Part model, mm, in its own coordinate system. Face numbers are marked on the shaded views. Round coordinates to 2 decimals unless told otherwise and drop trailing zeros. Loops run counter-clockwise (first coordinate to the right, second up) from the corner with the lowest first, then second, coordinate; pieces in that order, holes last. Notation, with made-up numbers: M 15.5,-4 L 43.5,-4 A23 ccw 43.5,14 Z; hole C 38,57 d6. An arc over 180 degrees is marked long. Answer as CSV lines item,"result". Start each with the question number.
Item 1: Drop a flat-ended pin along its axis: pin 1 Ø1.5 at (y, z) = (-2, 43.5) entering from -X. Give the stop position or say it passes through.
Item 2: Wall check: line 1 (Z direction, x = 17.5, y = -1.1); line 2 (Z direction, x = 16.25, y = -2.35); line 3 (X direction, y = -2.4, z = 23). Give the ranges that are in metal, low to high.
Item 3: Band-saw the part on A-A (y = -2.1). Give the cut face in (x, z).
Item 4: Mould opens along Y. For the marked faces 1 and 2 say: pulls with the +Y half, pulls with the -Y half, needs draft (parallel to the pull), parting line crosses it, or undercut.
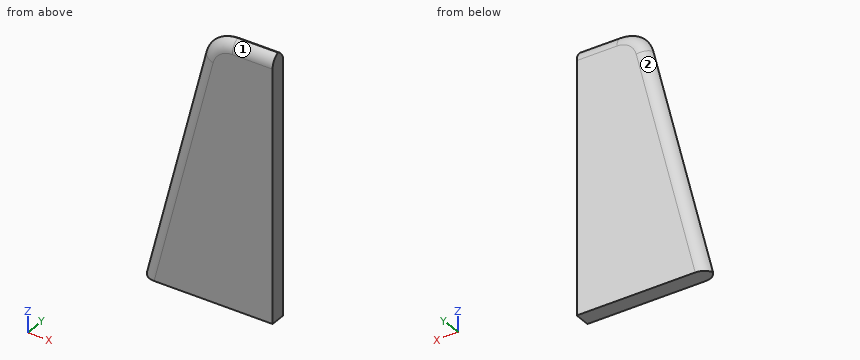
```python
from build123d import *

# Parameters (mm, degrees)
F1_DEPTH    = 3.048
F2_T1_DEPTH = 53.7555112647
F2_T3_DEPTH = 14.0920698193
F2_T6_ANGLE = 75.9637565321
F2_T8_ANGLE = 75.9637565321


# Not quite as in the source:
# - a fillet or chamfer that OpenCascade refuses, or shapes differently, is made with other operations: its cross-section is extruded or revolved along the edge and cut away or added


with BuildPart() as f1:
    # F0 (on Front) → F1 (new body)
    with BuildSketch(Plane.XZ):
        with BuildLine():
            Line((25.4, 50.8), (17.6579301807, 50.8))
            ThreePointArc((17.6579301807, 50.8), (13.750062651, 49.4551045314), (11.4975253047, 45.990101219))
            Line((11.4975253047, 45.990101219), (0, 0))
            Line((0, 0), (25.4, 0))
            Line((25.4, 0), (25.4, 50.8))
        make_face()
    extrude(amount=F1_DEPTH)

    # F2: fillet of radius 2.54 on 2 edges, made by hand

    # F2_s2 → F2_t1 (cut)
    with BuildSketch(Plane(origin=(11.4975253047, 0, 45.990101219), x_dir=(0, 1, 0), z_dir=(-0.242535625, 0, -0.9701425001))):
        with BuildLine():
            ThreePointArc((-0.508, 0), (-2.3040512242, 0.7439487758), (-3.048, 2.54))
            Line((-3.048, 2.54), (-3.048, 0))
            Line((-3.048, 0), (-0.508, 0))
        make_face()
        with BuildLine():
            ThreePointArc((-2.54, 0), (-0.7439487758, 0.7439487758), (0, 2.54))
            Line((0, 2.54), (0, 0))
            Line((0, 0), (-2.54, 0))
        make_face()
    extrude(amount=F2_T1_DEPTH, mode=Mode.SUBTRACT)

    # F2_s4 → F2_t3 (cut)
    with BuildSketch(Plane.YZ.offset(17.6579301807)):
        with BuildLine():
            ThreePointArc((-2.54, 50.8), (-0.7439487758, 50.0560512242), (0, 48.26))
            Line((0, 48.26), (0, 50.8))
            Line((0, 50.8), (-2.54, 50.8))
        make_face()
        with BuildLine():
            ThreePointArc((-0.508, 50.8), (-2.3040512242, 50.0560512242), (-3.048, 48.26))
            Line((-3.048, 48.26), (-3.048, 50.8))
            Line((-3.048, 50.8), (-0.508, 50.8))
        make_face()
    extrude(amount=F2_T3_DEPTH, mode=Mode.SUBTRACT)

    # F2_s5 → F2_t6 (revolve, cut)
    with BuildSketch(Plane.YZ.offset(17.6579301807)):
        with BuildLine():
            ThreePointArc((-2.54, 50.8), (-0.7439487758, 50.0560512242), (0, 48.26))
            Line((0, 48.26), (0, 50.8))
            Line((0, 50.8), (-2.54, 50.8))
        make_face()
    revolve(axis=Axis((17.6579301807, 0, 44.45), (0, -1, 0)), revolution_arc=F2_T6_ANGLE, mode=Mode.SUBTRACT)

    # F2_s7 → F2_t8 (revolve, cut)
    with BuildSketch(Plane.YZ.offset(17.6579301807)):
        with BuildLine():
            ThreePointArc((-0.508, 50.8), (-2.3040512242, 50.0560512242), (-3.048, 48.26))
            Line((-3.048, 48.26), (-3.048, 50.8))
            Line((-3.048, 50.8), (-0.508, 50.8))
        make_face()
    revolve(axis=Axis((17.6579301807, -3.048, 44.45), (0, -1, 0)), revolution_arc=F2_T8_ANGLE, mode=Mode.SUBTRACT)


solid = f1.part
```
Answer block:
1,pin 1,"stops at x = 10.95"
2,line 1,"z = 0 to 50.35"
2,line 2,"z = 0 to 49.83"
2,line 3,"x = 6.62 to 25.4"
3,outline,"M 0.58,0 L 25.4,0 L 25.4,50.24 L 17.66,50.24 A5.79 ccw 12.04,45.85 Z"
4,face 1,"pulls with the -Y half"
4,face 2,"pulls with the +Y half"
